Check sheet for the modelled part. Datum: model origin and axes. Units: mm. Face numbers are marked on the shaded views. Give positions to 0.01 mm unless a question says otherwise; leave off trailing zeros. Write each loop counter-clockwise with the first axis right and the second up, starting at its lowest first coordinate (ties: lowest second). Pieces come first, ordered by that corner, then holes.
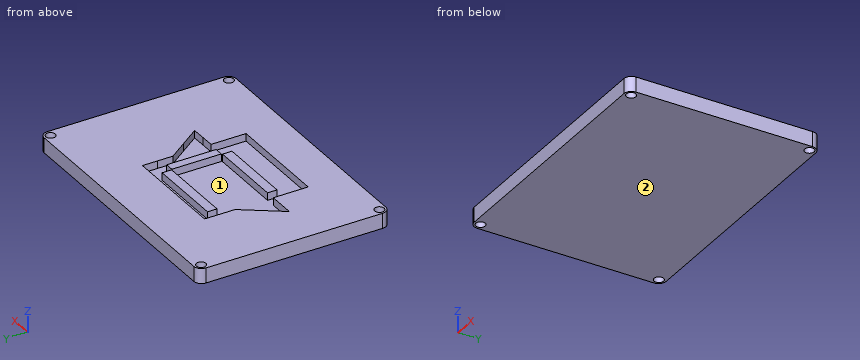
from build123d import *

# Parameters (mm, degrees)
SKETCH1_W            = 89.3572
SKETCH1_H            = 64.8208
SKETCH1_R            = 1.6
BOSS_EXTRUDE1_DEPTH  = 2.54
SKETCH2_W            = 89.3572
SKETCH2_H            = 64.8208
SKETCH2_R            = 1.6
BOSS_EXTRUDE11_DEPTH = 2.54
SKETCH3_W            = 2.92236531
SKETCH3_H            = 16.692
BOSS_EXTRUDE13_DEPTH = 2.54
FILLET1_R            = 2.54


with BuildPart() as part:
    # Sketch1 → Boss-Extrude1 (new body)
    with BuildSketch(Plane.XY):
        Rectangle(SKETCH1_W, SKETCH1_H)
        with Locations((-42.3926, 30.1244)):
            Circle(SKETCH1_R, mode=Mode.SUBTRACT)
        with Locations((-42.3926, -30.1244)):
            Circle(SKETCH1_R, mode=Mode.SUBTRACT)
        with Locations((42.3926, -30.1244)):
            Circle(SKETCH1_R, mode=Mode.SUBTRACT)
        with Locations((42.3926, 30.1244)):
            Circle(SKETCH1_R, mode=Mode.SUBTRACT)
    extrude(amount=BOSS_EXTRUDE1_DEPTH)

    # Sketch2 → Boss-Extrude11 (add)
    # profile 1 of 3: a face of its own
    with BuildSketch(Plane.XY.offset(2.54)):
        Rectangle(SKETCH2_W, SKETCH2_H)
        with Locations((42.3926, -30.1244)):
            Circle(SKETCH2_R, mode=Mode.SUBTRACT)
        with Locations((42.3926, 30.1244)):
            Circle(SKETCH2_R, mode=Mode.SUBTRACT)
        with Locations((-42.3926, -30.1244)):
            Circle(SKETCH2_R, mode=Mode.SUBTRACT)
        with Locations((-42.3926, 30.1244)):
            Circle(SKETCH2_R, mode=Mode.SUBTRACT)
        with BuildLine():
            add(Edge.make_bspline(
                [(-25.074263881, -0.273869479), (-27.394283412, -3.573869479), (-29.434224819, -6.473869479), (-29.594283412, -6.713908542)],
                knots=[18, 18, 18, 18, 19, 19, 19, 19], degree=3))
            Line((-29.594283412, -6.713908542), (-29.894283412, -7.173869479))
            Line((-29.894283412, -7.173869479), (-25.374263881, -7.173869479))
            Line((-25.374263881, -7.173869479), (-20.85424435, -7.173869479))
            Line((-20.85424435, -7.173869479), (-20.85424435, -13.073869479))
            Line((-20.85424435, -13.073869479), (-20.85424435, -18.973869479))
            Line((-20.85424435, -18.973869479), (-3.35424435, -18.973869479))
            Line((-3.35424435, -18.973869479), (14.14575565, -18.973869479))
            Line((14.14575565, -18.973869479), (14.14575565, -13.073869479))
            Line((14.14575565, -13.073869479), (14.14575565, -7.173869479))
            Line((14.14575565, -7.173869479), (18.705716588, -7.133830417))
            Line((18.705716588, -7.133830417), (23.285794713, -7.073869479))
            Line((23.285794713, -7.073869479), (18.725833775, -0.673869479))
            Line((18.725833775, -0.673869479), (14.165677525, 5.726130521))
            Line((14.165677525, 5.726130521), (14.14575565, 10.886091458))
            Line((14.14575565, 10.886091458), (14.14575565, 16.026130521))
            Line((14.14575565, 16.026130521), (-3.35424435, 16.026130521))
            Line((-3.35424435, 16.026130521), (-20.85424435, 16.026130521))
            Line((-20.85424435, 16.026130521), (-20.85424435, 10.866169583))
            Line((-20.85424435, 10.866169583), (-20.85424435, 5.726130521))
            Line((-20.85424435, 5.726130521), (-25.074263881, -0.273869479))
        make_face(mode=Mode.SUBTRACT)
    # profile 2 of 3: a face of its own
    with BuildSketch(Plane.XY.offset(2.54)):
        Polygon((-4.95424435, -7.173869479), (7.74575565, -7.173869479), (7.74575565, -8.773869479), (7.74575565, -10.373869479), (-4.95424435, -10.373869479), (-17.65424435, -10.373869479), (-17.65424435, -8.773869479), (-17.65424435, -7.173869479), align=None)
    # profile 3 of 3: a face of its own
    with BuildSketch(Plane.XY.offset(2.54)):
        Polygon((-17.85424435, 13.226130521), (-5.05424435, 13.226130521), (7.74575565, 13.226130521), (7.74575565, 11.626130521), (7.74575565, 10.026130521), (-5.05424435, 10.026130521), (-17.85424435, 10.026130521), (-17.85424435, 11.626130521), align=None)
    extrude(amount=BOSS_EXTRUDE11_DEPTH)

    # Sketch3 → Boss-Extrude13 (add)
    with BuildSketch(Plane.XY.offset(2.54)):
        with Locations((9.460938305, 1.426130521)):
            Rectangle(SKETCH3_W, SKETCH3_H)
    extrude(amount=BOSS_EXTRUDE13_DEPTH)

    # Fillet1
    fillet1_edges = [part.edges().sort_by_distance(p)[0] for p in [
        (-44.6786, 32.4104, 2.54),
        (44.6786, 32.4104, 2.54),
        (44.6786, -32.4104, 2.54),
        (-44.6786, -32.4104, 2.54),
    ]]
    fillet(fillet1_edges, radius=FILLET1_R)


solid = part.part
1) Sectioned sample at C-C on z = 4.05. Give the number of separate pieces and of enclosed holes in the cut face, then the cut area to 3 significant figures.
2) Scan lines: L1, parallel to X at y = 6.5, z = 4; L2, parallel to X at y = -2, z = 2.8; L3, parallel to X at y = -13.5, z = 2.9. Record each from-to range of solid material in increasing order.
3) Draft check along Y on the marked faces 1 and 2. Enter one of: +Y half, -Y half, draft (parallel to the pull), parting line (faces both ways), or undercut.
4) Sectioned sample at B-B on x = 9. Record the boundary of the cut face in (y, z).
5) Sectioned sample at A-A on y = -13.5. Record the boundary of the cut face in (x, z).
6) Sectioned sample at D-D on x = -3.5. Record the boundary of the cut face in (y, z), then the cut area to 3 significant figures.
Answers below:
1. separate pieces: 4
1. enclosed holes: 5
1. area: 4,620 mm2
2. L1: x = -44.68 to -20.85, 8 to 10.92, 14.16 to 44.68
2. L2: x = -44.68 to -26.29, 8 to 10.92, 19.67 to 44.68
2. L3: x = -44.68 to -20.85, 14.15 to 44.68
3. face 1: undercut
3. face 2: draft
4. outline: (-32.41, 0) - (32.41, 0) - (32.41, 5.08) - (16.03, 5.08) - (16.03, 2.54) - (9.77, 2.54) - (9.77, 5.08) - (-6.92, 5.08) - (-6.92, 2.54) - (-18.97, 2.54) - (-18.97, 5.08) - (-32.41, 5.08) - close
5. outline: (-44.68, 0) - (44.68, 0) - (44.68, 5.08) - (14.15, 5.08) - (14.15, 2.54) - (-20.85, 2.54) - (-20.85, 5.08) - (-44.68, 5.08) - close
6. outline: (-32.41, 0) - (32.41, 0) - (32.41, 5.08) - (16.03, 5.08) - (16.03, 2.54) - (13.23, 2.54) - (13.23, 5.08) - (10.03, 5.08) - (10.03, 2.54) - (-7.17, 2.54) - (-7.17, 5.08) - (-10.37, 5.08) - (-10.37, 2.54) - (-18.97, 2.54) - (-18.97, 5.08) - (-32.41, 5.08) - close
6. area: 257 mm2
